Here's the drawing with two shaded views (mm, measured from the low corner). I have some questions. Round coordinates to 2 decimals unless told otherwise and drop trailing zeros. Loops run counter-clockwise (first coordinate to the right, second up) from the corner with the lowest first, then second, coordinate; pieces in that order, holes last. Notation, with made-up numbers: M -25,45 L 4,45 A26 ccw 4,73 Z; hole C 79.5,-7 d5. An arc over 180 degrees is marked long. One line per item, written item: value. Start each with the question number.
Q1. Imagine slicing it at C-C (x = 27.25). Please give me the cut outline in (y, z).
Q2. Imagine slicing it at D-D (y = 20). Please give me the cut outline in (x, z), then the cut area to 4 significant figures.
Q3. Imagine slicing it at B-B (x = 101.25). Please give me the cut outline in (y, z).
Q4. Imagine slicing it at A-A (y = 69.5). Please give me the cut outline in (x, z), then the cut area to 3 significant figures.
Q5. Thinking about a two-plate mould opening in Y: for the marked faces 1, 2 and 3, which applies, released by +Y, released by -Y, zero draft, split by the parting line, or undercut?
Q6. I'm going to push flat-ended pins straight in: pin 1 Ø1.5 at (x, y) = (91.5, 39) entering from +Z; pin 2 Ø7 at (x, y) = (27.25, 69.5) entering from -Z; pin 3 Ø3 at (x, y) = (28, 69.5) entering from +Z. Where does each tip first touch, or does it pass through?
Q7. Please list where these lines run through material, in increasing order: line 1 along Y through (x, z) = (27.25, 3.5); line 2 along Y through (x, z) = (101.25, 1.2); line 3 along X through (y, z) = (69.5, 1).
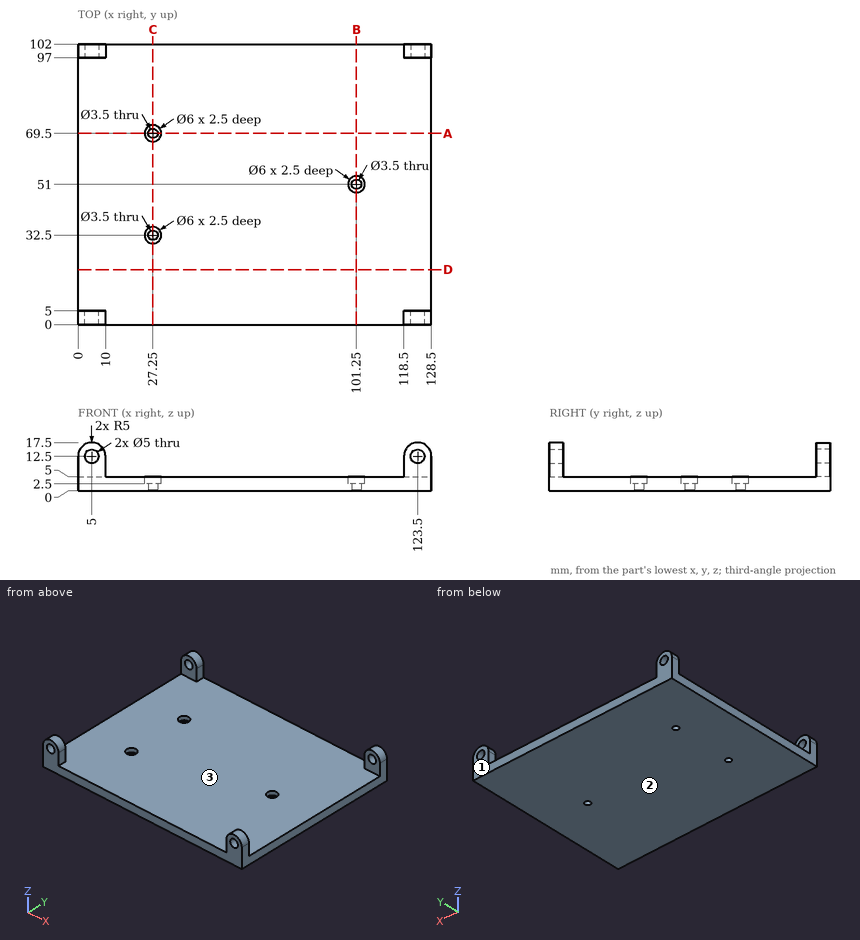
Report:
1. outline: M 0,0 L 30.75,0 L 30.75,2.5 L 29.5,2.5 L 29.5,5 L 0,5 Z; M 34.25,0 L 67.75,0 L 67.75,2.5 L 66.5,2.5 L 66.5,5 L 35.5,5 L 35.5,2.5 L 34.25,2.5 Z; M 71.25,0 L 102,0 L 102,5 L 72.5,5 L 72.5,2.5 L 71.25,2.5 Z
2. outline: M 0,0 L 128.5,0 L 128.5,5 L 0,5 Z
2. area: 642.5 mm²
3. outline: M 0,0 L 49.25,0 L 49.25,2.5 L 48,2.5 L 48,5 L 0,5 Z; M 52.75,0 L 102,0 L 102,5 L 54,5 L 54,2.5 L 52.75,2.5 Z
4. outline: M 0,0 L 25.5,0 L 25.5,2.5 L 24.25,2.5 L 24.25,5 L 0,5 Z; M 29,0 L 128.5,0 L 128.5,5 L 30.25,5 L 30.25,2.5 L 29,2.5 Z
4. area: 619 mm²
5. face 1: released by +Y
5. face 2: zero draft
5. face 3: undercut
6. pin 1: stops at z = 5
6. pin 2: stops at z = 0
6. pin 3: stops at z = 2.5
7. line 1: y = 0 to 29.5, 35.5 to 66.5, 72.5 to 102
7. line 2: y = 0 to 49.25, 52.75 to 102
7. line 3: x = 0 to 25.5, 29 to 128.5
